For this review, take the finished solid that the model builds, in its own axes (mm). A direction names the side the tool comes from. Coordinates: 2 decimals unless noted, no trailing zeros. Loops run counter-clockwise (first coordinate to the right, second up) from the corner with the lowest first, then second, coordinate; pieces in that order, holes last. Notation, with made-up numbers: (68, 17) - (102, 17) arc R31 ccw to (102, 56) - close; hole circle Ø4 at (-17, -32.5). An arc over 180 degrees is marked (long way). Answer as a JSON object with one key per item and string values. Group by question number.
Item 1: Clearance check with a flat-ended pin moving along its axis: pin 1 (1 mm diameter, centred on y = -8, z = 1.5, fed in from +X). State where the tip first meets the part, or that it passes through.
Item 2: To check wall thickness, follow line 1 (Y direction, x = 0, z = 2.3); line 2 (X direction, y = -1, z = 0.75); line 3 (Y direction, x = 31, z = 0.75). State the ranges of each line that lie inside material, in increasing order.
Item 3: We need section C-C (x = 62). Give the boundary of the cut face in (y, z), then the cut area to 3 significant figures.
Item 4: We need section B-B (x = 196). Give the boundary of the cut face in (y, z), then the cut area to 3 significant figures.
Item 5: We need section D-D (y = 13). Give the boundary of the cut face in (x, z).
Item 6: Mouldability with a two-part tool opening along X and no side actions: class faces 3 (the flat face through (206.722, 4.982, 1.479)), 4 (the flat face through (196.23, -27.38, 1.48)), 5 (the flat face through (132, 0, 0)) as released by +X, released by -X, zero draft, split by the parting line, or undercut.
Item 7: We need section A-A (z = 1.85). Give the boundary of the cut face in (x, y).
Item 8: Tool access review of faces 1 (the flat face through (133.99, -26.01, 1.48)), 2 (the flat face through (152.613, 5.313, 1.521)): name each direction out of +Z, -Z, +X, -X, +Y, -Y from which nothing blocks a thin tool from reaching the whole face with its end or side.
from build123d import *

# Parameters (mm, degrees)
BOSS_EXTRUDE1_DEPTH = 3
SKETCH4_R           = 4
CUT_EXTRUDE1_DEPTH  = 3
FILLET1_R           = 3
FILLET2_R           = 3
FILLET4_R           = 3
FILLET5_R           = 3


with BuildPart() as part:
    # Sketch3 → Boss-Extrude1 (new body)
    with BuildSketch(Plane.XY):
        with BuildLine():
            Line((90, 10), (0, 10))
            ThreePointArc((0, 10), (-10, 0), (0, -10))
            Line((0, -10), (89.999342556, -10))
            Line((89.999342556, -10), (179.234195732, -42.478830415))
            ThreePointArc((179.234195732, -42.478830415), (198.912530475, -43.888338079), (216.37877505, -34.714796202))
            Line((216.37877505, -34.714796202), (177.783610295, -20.667305045))
            Line((177.783610295, -20.667305045), (189.412295169, 11.282244062))
            Line((189.412295169, 11.282244062), (227, -2.398561671))
            ThreePointArc((227, -2.398561671), (212.1956726, 20.839577528), (185.295586496, 26.803183042))
            Line((185.295586496, 26.803183042), (90, 10))
        make_face()
    extrude(amount=BOSS_EXTRUDE1_DEPTH)

    # Sketch4 → Cut-Extrude1 (cut)
    with BuildSketch(Plane.XY.offset(3)):
        Circle(SKETCH4_R)
        Polygon((157.937239429, -10.553104382), (158.016476937, 2.148354383), (147.056309736, 8.56770546), (136.016905026, 2.285597773), (135.937667518, -10.415860992), (146.897834719, -16.835212069), align=None)
    extrude(amount=-CUT_EXTRUDE1_DEPTH, mode=Mode.SUBTRACT)

    # Fillet1
    fillet1_edges = [part.edges().sort_by_distance(p)[0] for p in [
        (177.783610295, -20.667305045, 1.5),
    ]]
    fillet(fillet1_edges, radius=FILLET1_R)

    # Fillet2
    fillet2_edges = [part.edges().sort_by_distance(p)[0] for p in [
        (189.412295169, 11.282244062, 1.5),
    ]]
    fillet(fillet2_edges, radius=FILLET2_R)

    # Fillet4
    fillet4_edges = [part.edges().sort_by_distance(p)[0] for p in [
        (227, -2.398561671, 1.5),
    ]]
    fillet(fillet4_edges, radius=FILLET4_R)

    # Fillet5
    fillet5_edges = [part.edges().sort_by_distance(p)[0] for p in [
        (216.37877505, -34.714796202, 1.5),
    ]]
    fillet(fillet5_edges, radius=FILLET5_R)


solid = part.part
Check sheet entries:
{
 "1": {"pin 1": "stops at x = 182.58"},
 "2": {"line 1": "y = -10 to -4, 4 to 10", "line 2": "x = -9.95 to -3.87, 3.87 to 136, 158 to 184.94", "line 3": "y = -10 to 10"},
 "3": {"outline": "(-10, 0) - (10, 0) - (10, 3) - (-10, 3) - close", "area": "60.0 mm2"},
 "4": {"outline": "(-44.37, 0) - (-27.3, 0) - (-27.3, 3) - (-44.37, 3) - close; (8.88, 0) - (27.07, 0) - (27.07, 3) - (8.88, 3) - close", "area": "106 mm2"},
 "5": {"outline": "(107.01, 0) - (220.31, 0) - (220.31, 3) - (107.01, 3) - close"},
 "6": {"face 3": "undercut", "face 4": "released by +X", "face 5": "zero draft"},
 "7": {"outline": "(0, -10) - (90, -10) - (179.23, -42.48) arc R36 ccw to (212.12, -38.19) arc R3 ccw to (211.43, -32.91) - (180.6, -21.69) arc R3 cw to (178.81, -17.85) - (188.39, 8.46) arc R3 cw to (192.23, 10.26) - (221.62, -0.44) arc R3 ccw to (225.48, 3.38) arc R36 ccw to (185.3, 26.8) - (90, 10) - (0, 10) arc R10 ccw to start; hole circle Ø8 at (0, 0); hole (135.94, -10.42) - (146.9, -16.84) - (157.94, -10.55) - (158.02, 2.15) - (147.06, 8.57) - (136.02, 2.29) - close"},
 "8": {"face 1": "+Z, -Z, -X, -Y", "face 2": "+Z, -Z"}
}
